Input: dimensioned drawing with shaded views. Units: mm. Origin: part minimum x, y, z. Give positions to 0.01 mm unless a question says otherwise; leave off trailing zeros. Loops run counter-clockwise (first coordinate to the right, second up) from the corner with the lowest first, then second, coordinate; pieces in that order, holes last.
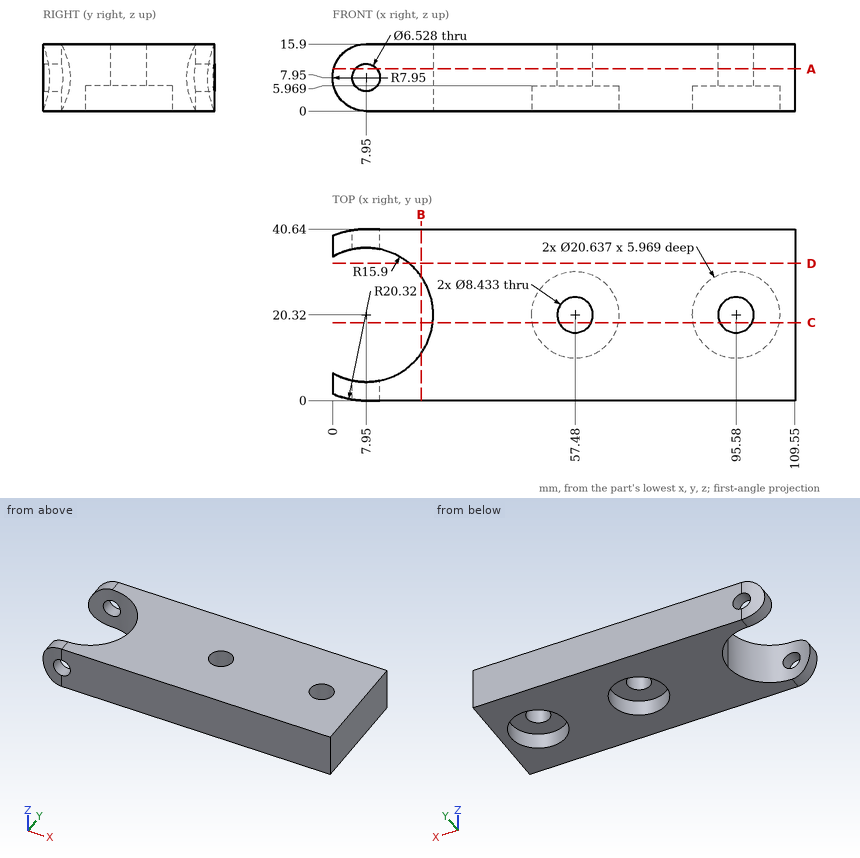
(1) Ray query, line 1 along X through (y, z) = (17, 5.25); line 2 along Y through (x, z) = (97, 13.75); line 3 along Y through (x, z) = (20.5, 4.5) (1 decimal). Return the intervals inside material, ascending.
A:
line 1: x = 23.5 to 47.71, 67.25 to 85.81, 105.35 to 109.55
line 2: y = 0 to 16.35, 24.29 to 40.64
line 3: y = 0 to 10.6, 30.1 to 40.6
(2) Section A-A, the plane z = 10. Return the cut outline in (x, y), then the cut area to 4 significant figures.
A:
outline: (0.27, 1.51) arc R20.32 ccw to (5.41, 0.16) - (5.41, 4.62) arc R15.9 cw to (0.27, 6.4) - close; (0.27, 34.24) arc R15.9 cw to (5.41, 36.02) - (5.41, 40.48) arc R20.32 ccw to (0.27, 39.13) - close; (10.49, 0) - (109.55, 0) - (109.55, 40.64) - (10.49, 40.64) - (10.49, 36.02) arc R15.9 cw to (10.49, 4.62) - close; hole circle Ø8.43 at (57.48, 20.32); hole circle Ø8.43 at (95.58, 20.32)
area: 3,645 mm2
(3) Section C-C, the plane y = 18.5. Return the cut outline in (x, z).
A:
outline: (23.75, 0) - (47.32, 0) - (47.32, 5.97) - (53.68, 5.97) - (53.68, 15.9) - (23.75, 15.9) - close; (61.28, 5.97) - (67.64, 5.97) - (67.64, 0) - (85.42, 0) - (85.42, 5.97) - (91.78, 5.97) - (91.78, 15.9) - (61.28, 15.9) - close; (99.38, 5.97) - (105.74, 5.97) - (105.74, 0) - (109.55, 0) - (109.55, 15.9) - (99.38, 15.9) - close
(4) Section B-B, the plane x = 21. Return the cut outline in (y, z) (1 decimal).
A:
outline: (0, 0) - (11.2, 0) - (11.2, 15.9) - (0, 15.9) - close; (29.4, 0) - (40.6, 0) - (40.6, 15.9) - (29.4, 15.9) - close
(5) Section D-D, the plane y = 32.5. Return the cut outline in (x, z), then the cut area to 3 significant figures.
A:
outline: (18.17, 0) - (109.55, 0) - (109.55, 15.9) - (18.17, 15.9) - close
area: 1,450 mm2
(6) First-contact query: pin 1 (6 mm diameter, centred on x = 7.95, z = 7.95, fed in from +Y); pin 2 (1 mm diameter, centred on y = 9, z = 12.5, fed in from -X) (1 decimal); pin 3 (1.5 mm diameter, centred on y = 35.5, z = 4.5, fed in from -X); pin 4 (6 mm diameter, centred on x = 98.5, y = 17.5, fed in from -Z). Flat tips, straight axial feed; report the tip coordinate or a pass-through.
A:
pin 1: passes through
pin 2: stops at x = 18.6
pin 3: stops at x = 0.47
pin 4: stops at z = 5.97
